The listing builds one solid part. Answer for the finished solid, in the listing's coordinates (mm). A direction names the side the tool comes from. Round coordinates to 2 decimals unless told otherwise and drop trailing zeros. Loops run counter-clockwise (first coordinate to the right, second up) from the corner with the lowest first, then second, coordinate; pieces in that order, holes last. Notation, with made-up numbers: (59.25, 51.5) -> (102.25, 51.5) arc R21 cw to (102.25, 76.5) -> close; hole circle Ø7 at (-28, -11). An arc over 180 degrees is marked (long way). One line per question, with ' | ' between items.
from build123d import *

# Parameters (mm, degrees)
F0_W            = 20
F0_H            = 30
F1_DEPTH        = 9
F4_W            = 10.2
F4_H            = 13
F5_DEPTH        = 7
F2_W            = 4
F2_H            = 30
F6_DEPTH        = 15
F7_R            = 6
F10_D           = 4.1
F10_CSINK_D     = 8.5
F10_CSINK_ANGLE = 90
F11_F1_R        = 5
F11_F2_R        = 5
F11_T3_DEPTH    = 20
F11_T5_DEPTH    = 16.5
F11_T8_ANGLE    = 90
F11_T10_ANGLE   = 90
F11_T11_DEPTH   = 20
F11_T13_DEPTH   = 31.5
F11_T16_ANGLE   = 90
F11_T18_ANGLE   = 90
F13_T1_DEPTH    = 40


# Not quite as in the source:
# - a fillet or chamfer that OpenCascade refuses, or shapes differently, is made with other operations: its cross-section is extruded or revolved along the edge and cut away or added
# - a feature of the source that left no trace in its solid (it failed there, or was rolled back) is left out


with BuildPart() as f1:
    # F0 (on Top) → F1 (new body)
    with BuildSketch(Plane.XY):
        with Locations((-10, 15)):
            Rectangle(F0_W, F0_H)
    extrude(amount=F1_DEPTH)

    # F4 (on offset) → F5 (cut)
    with BuildSketch(Plane.XY.offset(9)):
        with Locations((-10, 16.5)):
            Rectangle(F4_W, F4_H)
    extrude(amount=-F5_DEPTH, mode=Mode.SUBTRACT)

    # F2 (on Top) → F6 (join)
    with BuildSketch(Plane.XY):
        with Locations((-2, 15)):
            Rectangle(F2_W, F2_H)
    extrude(amount=-F6_DEPTH)

    # F7
    f7_edges = [f1.edges().sort_by_distance(p)[0] for p in [
        (-10, 10, 2),
        (-10, 23, 2),
    ]]
    fillet(f7_edges, radius=F7_R)

    # F10 (through all)
    with Locations(Plane.YZ):
        with Locations((7, -8.5), (23, -8.5)):
            CounterSinkHole(F10_D / 2, F10_CSINK_D / 2, counter_sink_angle=F10_CSINK_ANGLE)

    # F11: fillet of radius 5 on 4 edges, made by hand

    # F11_f1
    f11_f1_edges = [f1.edges().sort_by_distance(p)[0] for p in [
        (-10, 0, 9),
    ]]
    fillet(f11_f1_edges, radius=F11_F1_R)

    # F11_f2
    f11_f2_edges = [f1.edges().sort_by_distance(p)[0] for p in [
        (-10, 30, 9),
    ]]
    fillet(f11_f2_edges, radius=F11_F2_R)

    # F11_s4 → F11_t3 (cut)
    with BuildSketch(Plane.XZ.offset(-25)):
        with BuildLine():
            ThreePointArc((-15, 9), (-18.5355339059, 7.5355339059), (-20, 4))
            Line((-20, 4), (-20.1, 4))
            Line((-20.1, 4), (-20.1, 9.1))
            Line((-20.1, 9.1), (-15, 9.1))
            Line((-15, 9.1), (-15, 9))
        make_face()
    extrude(amount=F11_T3_DEPTH, mode=Mode.SUBTRACT)

    # F11_s6 → F11_t5 (cut)
    with BuildSketch(Plane.XY.offset(-12.5)):
        with BuildLine():
            ThreePointArc((-20, 5), (-18.5355339059, 1.4644660941), (-15, 0))
            Line((-15, 0), (-15, -0.1))
            Line((-15, -0.1), (-20.1, -0.1))
            Line((-20.1, -0.1), (-20.1, 5))
            Line((-20.1, 5), (-20, 5))
        make_face()
        with BuildLine():
            ThreePointArc((-20, 25), (-18.5355339059, 28.5355339059), (-15, 30))
            Line((-15, 30), (-15, 30.1))
            Line((-15, 30.1), (-20.1, 30.1))
            Line((-20.1, 30.1), (-20.1, 25))
            Line((-20.1, 25), (-20, 25))
        make_face()
    extrude(amount=F11_T5_DEPTH, mode=Mode.SUBTRACT)

    # F11_s7 → F11_t8 (revolve, cut)
    with BuildSketch(Plane.XZ.offset(-25)):
        with BuildLine():
            ThreePointArc((-20, 4), (-18.5355339059, 7.5355339059), (-15, 9))
            Line((-15, 9), (-15, 9.1))
            Line((-15, 9.1), (-20.1, 9.1))
            Line((-20.1, 9.1), (-20.1, 4))
            Line((-20.1, 4), (-20, 4))
        make_face()
    revolve(axis=Axis((-20, 25, 4), (-1, 0, 0)), revolution_arc=F11_T8_ANGLE, mode=Mode.SUBTRACT)

    # F11_s9 → F11_t10 (revolve, cut)
    with BuildSketch(Plane.XZ.offset(-5)):
        with BuildLine():
            ThreePointArc((-20, 4), (-18.5355339059, 7.5355339059), (-15, 9))
            Line((-15, 9), (-15, 9.1))
            Line((-15, 9.1), (-20.1, 9.1))
            Line((-20.1, 9.1), (-20.1, 4))
            Line((-20.1, 4), (-20, 4))
        make_face()
    revolve(axis=Axis((-20, 5, 4), (1, 0, 0)), revolution_arc=F11_T10_ANGLE, mode=Mode.SUBTRACT)

    # F11_s12 → F11_t11 (cut)
    with BuildSketch(Plane.XZ.offset(-25)):
        with BuildLine():
            ThreePointArc((-5, 9), (-1.4644660941, 7.5355339059), (0, 4))
            Line((0, 4), (0.1, 4))
            Line((0.1, 4), (0.1, 9.1))
            Line((0.1, 9.1), (-5, 9.1))
            Line((-5, 9.1), (-5, 9))
        make_face()
    extrude(amount=F11_T11_DEPTH, mode=Mode.SUBTRACT)

    # F11_s14 → F11_t13 (cut)
    with BuildSketch(Plane.XY.offset(-27.5)):
        with BuildLine():
            ThreePointArc((0, 25), (-1.4644660941, 28.5355339059), (-5, 30))
            Line((-5, 30), (-5, 30.1))
            Line((-5, 30.1), (0.1, 30.1))
            Line((0.1, 30.1), (0.1, 25))
            Line((0.1, 25), (0, 25))
        make_face()
        with BuildLine():
            ThreePointArc((0, 5), (-1.4644660941, 1.4644660941), (-5, 0))
            Line((-5, 0), (-5, -0.1))
            Line((-5, -0.1), (0.1, -0.1))
            Line((0.1, -0.1), (0.1, 5))
            Line((0.1, 5), (0, 5))
        make_face()
    extrude(amount=F11_T13_DEPTH, mode=Mode.SUBTRACT)

    # F11_s15 → F11_t16 (revolve, cut)
    with BuildSketch(Plane.XZ.offset(-5)):
        with BuildLine():
            ThreePointArc((0, 4), (-1.4644660941, 7.5355339059), (-5, 9))
            Line((-5, 9), (-5, 9.1))
            Line((-5, 9.1), (0.1, 9.1))
            Line((0.1, 9.1), (0.1, 4))
            Line((0.1, 4), (0, 4))
        make_face()
    revolve(axis=Axis((0, 5, 4), (1, 0, 0)), revolution_arc=F11_T16_ANGLE, mode=Mode.SUBTRACT)

    # F11_s17 → F11_t18 (revolve, cut)
    with BuildSketch(Plane.XZ.offset(-25)):
        with BuildLine():
            ThreePointArc((-5, 9), (-1.4644660941, 7.5355339059), (0, 4))
            Line((0, 4), (0.1, 4))
            Line((0.1, 4), (0.1, 9.1))
            Line((0.1, 9.1), (-5, 9.1))
            Line((-5, 9.1), (-5, 9))
        make_face()
    revolve(axis=Axis((0, 25, 4), (-1, 0, 0)), revolution_arc=F11_T18_ANGLE, mode=Mode.SUBTRACT)

    # F13: fillet of radius 4 on 1 edges, made by hand

    # F13_s2 → F13_t1 (cut)
    with BuildSketch(Plane.XZ.offset(-35)):
        with BuildLine():
            ThreePointArc((0, -11), (-1.1715728753, -13.8284271247), (-4, -15))
            Line((-4, -15), (0, -15))
            Line((0, -15), (0, -11))
        make_face()
    extrude(amount=F13_T1_DEPTH, mode=Mode.SUBTRACT)


solid = f1.part
Q1. Find the intervals of material crossed by line 1 (Y direction, x = -3.25, z = -8.5); line 2 (Y direction, x = -2.9, z = -8.5); line 3 (Z direction, x = -2.7, y = 7), in increasing order. Write a range as from..to.
Numbers:
line 1: 0.32..4.95, 9.05..20.95, 25.05..29.68 | line 2: 0.46..4.95, 9.05..20.95, 25.05..29.54 | line 3: -14.78..-10.55, -6.45..8.44
Q2. A cutting plane is placed at B-B on x = -13.25. Give the vertices of the cut face in (y, z).
Numbers:
outline: (0, 0) -> (30, 0) -> (30, 4) arc R5 ccw to (25, 9) -> (23, 9) -> (23, 8) arc R6 cw to (17, 2) -> (16, 2) arc R6 cw to (10, 8) -> (10, 9) -> (5, 9) arc R5 ccw to (0, 4) -> close
Q3. A cutting plane is placed at C-C on z = -8.5. Give the vertices of the cut face in (x, y).
Numbers:
outline: (-4, 0.1) arc R5 ccw to (-0.37, 3.12) -> (-2.2, 4.95) -> (-4, 4.95) -> close; (-4, 9.05) -> (-2.2, 9.05) -> (0, 11.25) -> (0, 18.75) -> (-2.2, 20.95) -> (-4, 20.95) -> close; (-4, 25.05) -> (-2.2, 25.05) -> (-0.37, 26.88) arc R5 ccw to (-4, 29.9) -> close
Q4. A cutting plane is placed at A-A on y = 7. Give the vertices of the cut face in (x, z), plus the area to 3 significant figures.
Numbers:
outline: (-20, 0) -> (-4, 0) -> (-4, -6.45) -> (-2.2, -6.45) -> (0, -4.25) -> (0, 4) arc R5 ccw to (-5, 9) -> (-15, 9) arc R5 ccw to (-20, 4) -> close; (-4, -15) arc R4 ccw to (-0.28, -12.47) -> (-2.2, -10.55) -> (-4, -10.55) -> close | area: 205 mm^2
Q5. Given pin 1 Ø4 at (y, z) = (25.5, 2) entering from -X; pin 2 Ø6.5 at (y, z) = (23, -8.5) entering from +X; pin 3 Ø1.1 at (x, y) = (-8, 16.5) entering from +Z; pin 4 Ø3 at (x, y) = (-6, 17) entering from -Z, each flat-ended and moving along its own axis, determine where each tip first touches the part or whether it passes through.
Numbers:
pin 1: x = -20 | pin 2: x = -1 | pin 3: z = 2 | pin 4: z = 0
Q6. For a pull along X with two mould halves and no side action, classify faces 3 (the face through (-18, 15, 8)), 4 (the face through (-1, 28, -4)), 5 (the face through (-3.11, 25.05, -8.41)), 6 (the face through (-9.929, 21.196, 3.711)) as pulls with the +X half, pulls with the -X half, needs draft (parallel to the pull), parting line crosses it, or undercut.
Numbers:
face 3: pulls with the -X half | face 4: pulls with the +X half | face 5: needs draft | face 6: undercut
Q7. For faces 1 (the face through (-10, 8, 9)), 2 (the face through (-15.1, 16, 6)), determine the directions among +Z, -Z, +X, -X, +Y, -Y from which every point of the face is accessible in a straight line to the end or side of a thin tool.
Numbers:
face 1: +Z, +X, -X, +Y, -Y | face 2: +Z
Q8. A cutting plane is placed at D-D on y = 14. Give the vertices of the cut face in (x, z).
Numbers:
outline: (-20, 0) -> (-4, 0) -> (-4, -15) arc R4 ccw to (0, -11) -> (0, 4) arc R5 ccw to (-4.9, 9) -> (-4.9, 2.34) -> (-15.1, 2.34) -> (-15.1, 9) arc R5 ccw to (-20, 4) -> close
